```python
from build123d import *

# Parameters (mm, degrees)
EXTRUDE_START       = -2
SKETCH_1_R          = 15
SKETCH_1_R_2        = 4
EXTRUDE_1_DEPTH     = 4
SKETCH_2_R          = 2
CUT_EXTRUDE_1_DEPTH = 99.856382383


with BuildPart() as part:
    # Эскиз1 → Вытянуть1 (new body)
    with BuildSketch(Plane.XY.offset(EXTRUDE_START)):
        with BuildLine():
            Line((-81.676846175, 13.911980398), (-2.13800288, 29.923718748))
            ThreePointArc((-2.13800288, 29.923718748), (29.996326682, 0.469452404), (-1.200553025, -29.975968248))
            Line((-1.200553025, -29.975968248), (-81.702325517, -13.909086088))
            ThreePointArc((-81.702325517, -13.909086088), (-94.109421594, 0.012821602), (-81.676846175, 13.911980398))
        make_face()
        Circle(SKETCH_1_R, mode=Mode.SUBTRACT)
        with Locations((-81.917641848, 0)):
            Circle(SKETCH_1_R_2, mode=Mode.SUBTRACT)
    extrude(amount=EXTRUDE_1_DEPTH)

    # Эскиз2 → Вырез-Вытянуть1 (cut, through all)
    with BuildSketch(Plane.XY.offset(2)):
        with Locations((-17.747047674, -15.205235902)):
            Circle(SKETCH_2_R)
        with Locations((-23.247368562, 2.390973642)):
            Circle(SKETCH_2_R)
        with Locations((-14.694283668, 18.722686931)):
            Circle(SKETCH_2_R)
        with Locations((19.233639165, 15.669922925)):
            Circle(SKETCH_2_R)
        with Locations((24.733960053, -1.926286619)):
            Circle(SKETCH_2_R)
        with Locations((16.180875159, -18.257999908)):
            Circle(SKETCH_2_R)
    extrude(amount=-CUT_EXTRUDE_1_DEPTH, mode=Mode.SUBTRACT)


solid = part.part
```
Could you check a few things on this model? Use its own coordinates, in mm. Round coordinates to 2 decimals unless told otherwise and drop trailing zeros. Loops run counter-clockwise (first coordinate to the right, second up) from the corner with the lowest first, then second, coordinate; pieces in that order, holes last. Notation, with made-up numbers: M -32.5,35 L -7.5,35 A21 cw -7.5,60 Z; hole C 38,13 d4. An arc over 180 degrees is marked long. Answer as CSV lines item,"result".
1) If I drill on probe 1 along X at (y, z) = (-2.5, 0.1); probe 2 along Y at (x, z) = (0, 1); probe 3 along Y at (x, z) = (-22, -1.65), over which ranges is the centre line in solid material (lowest first)?
From the geometry:
probe 1,"-93.88 to -85.04, -78.8 to -14.79, 14.79 to 22.82, 26.65 to 29.9"
probe 2,"-30 to -15, 15 to 30"
probe 3,"-25.82 to 0.83, 3.95 to 25.93"
2) We'd pull the mould along X, two halves only. Please class faces 1 (the cylindrical face through (-14.985, 0.66, -0.028)), 2 (the flat face through (-31, 0, -2)), 3 (the flat face through (-42.5, 21.8, 0)): released by +X, released by -X, zero draft, split by the parting line, or undercut.
From the geometry:
face 1,"undercut"
face 2,"zero draft"
face 3,"released by -X"
3) Imagine slicing it at C-C on z = -0.5. Count the separate pieces of the cut face and the enclosed holes in it, and give its area (3 significant figures).
From the geometry:
separate pieces,"1"
enclosed holes,"8"
area,"4,450 mm^2"
4) Imagine slicing it at A-A on x = 0. List the corners of the cut face in (y, z) for me, and give its area (3 significant figures).
From the geometry:
outline,"M -30,-2 L -15,-2 L -15,2 L -30,2 Z; M 15,-2 L 30,-2 L 30,2 L 15,2 Z"
area,"120 mm^2"
5) Imagine slicing it at B-B on y = -5.5. List the corners of the cut face in (x, z) for me.
From the geometry:
outline,"M -92.98,-2 L -13.96,-2 L -13.96,2 L -92.98,2 Z; M 13.96,-2 L 29.49,-2 L 29.49,2 L 13.96,2 Z"
6) Imagine slicing it at D-D on x = -58. List the corners of the cut face in (y, z) for me, and give its area (3 significant figures).
From the geometry:
outline,"M -18.64,-2 L 18.68,-2 L 18.68,2 L -18.64,2 Z"
area,"149 mm^2"
7) For pin 1 Ø1 at (x, z) = (-55, -0.5) entering from -Y; pin 2 Ø6.5 at (x, y) = (19.23, 15.67) entering from +Z; pin 3 Ø6 at (x, y) = (-69, 22) entering from -Z; pin 4 Ø1 at (x, z) = (-19, 1) entering from -Y, each with a flat end and sliding along its axis, tell me the tip position at first contact or that it passes through.
From the geometry:
pin 1,"y = -19.34"
pin 2,"z = 2"
pin 3,"through"
pin 4,"y = -26.52"
